For this review, take the finished solid that the model builds, in its own axes (mm). A direction names the side the tool comes from. Coordinates: 2 decimals unless noted, no trailing zeros. Loops run counter-clockwise (first coordinate to the right, second up) from the corner with the lowest first, then second, coordinate; pieces in that order, holes last. Notation, with made-up numbers: M 7,83 L 37,83 A20 ccw 37,94 Z; hole C 75.5,64.25 d1. An arc over 180 degrees is marked long. Write item = value, one per line.
from build123d import *

# Parameters (mm, degrees)
BOSS_EXTRUDE1_DEPTH = 25
SKETCH2_R           = 4
SKETCH2_R_2         = 1.5
CUT_EXTRUDE1_DEPTH  = 69.271516755
SKETCH3_R           = 4
SKETCH3_R_2         = 1.5
CUT_EXTRUDE2_DEPTH  = 71.774289117


with BuildPart() as part:
    # Sketch1 → Boss-Extrude1 (new body)
    with BuildSketch(Plane.XY):
        Polygon((-26, 30), (-26, -28), (26, -28), (26, 30), (28, 30), (28, -30), (-28, -30), (-28, 30), align=None)
    extrude(amount=BOSS_EXTRUDE1_DEPTH)

    # Sketch2 → Cut-Extrude1 (cut, through all)
    with BuildSketch(Plane(origin=(28, 0, 0), x_dir=(0, 0, -1), z_dir=(1, 0, 0))):
        with Locations((-12.5, 17.5)):
            Circle(SKETCH2_R)
        with Locations((-19.5, 17.5)):
            Circle(SKETCH2_R_2)
        with Locations((-12.5, -1.5)):
            Circle(SKETCH2_R_2)
        with Locations((-12.5, -18.5)):
            Circle(SKETCH2_R_2)
        with Locations((-12.5, 24.5)):
            Circle(SKETCH2_R_2)
        with Locations((-5.5, 17.5)):
            Circle(SKETCH2_R_2)
        with Locations((-12.5, 10.5)):
            Circle(SKETCH2_R_2)
        with BuildLine():
            Line((-25, 17.5), (-25, 33.655619926))
            Line((-25, 33.655619926), (0, 33.655619926))
            Line((0, 33.655619926), (0, 17.5))
            ThreePointArc((0, 17.5), (-12.5, 30), (-25, 17.5))
        make_face()
    extrude(amount=-CUT_EXTRUDE1_DEPTH, mode=Mode.SUBTRACT)

    # Sketch3 → Cut-Extrude2 (cut, through all)
    with BuildSketch(Plane.XZ.offset(30)):
        with Locations(Location((0, 12.5, 0), (0, 0, 270))):
            Circle(SKETCH3_R)
        with Locations(Location((-7, 12.5, 0), (0, 0, 270))):
            Circle(SKETCH3_R_2)
        with Locations(Location((0, 19.5, 0), (0, 0, 270))):
            Circle(SKETCH3_R_2)
        with Locations(Location((7, 12.5, 0), (0, 0, 270))):
            Circle(SKETCH3_R_2)
        with Locations(Location((0, 5.5, 0), (0, 0, 270))):
            Circle(SKETCH3_R_2)
        with Locations(Location((-19, 12.5, 0), (0, 0, 270))):
            Circle(SKETCH3_R_2)
        with Locations(Location((19, 12.5, 0), (0, 0, 270))):
            Circle(SKETCH3_R_2)
    extrude(amount=-CUT_EXTRUDE2_DEPTH, mode=Mode.SUBTRACT)


solid = part.part
Q1. For line 1 along X through (y, z) = (-28.55, 12.5); line 2 along Y through (x, z) = (-26.75, 12.5); line 3 along X through (y, z) = (10.5, 19.5), list the stretches that pass through material, from the lowest coordinate up.
Solved:
line_1 = -28 to -20.5, -17.5 to -8.5, -5.5 to -4, 4 to 5.5, 8.5 to 17.5, 20.5 to 28
line_2 = -30 to -20, -17 to -3, 0 to 9, 12 to 13.5, 21.5 to 23, 26 to 30
line_3 = -28 to -26, 26 to 28
Q2. Machinability: for faces 1 (the face through (27.014, 29.997, 12.225)), 2 (the face through (5, -28, 12)), which of the approach directions +Z, -Z, +X, -X, +Y, -Y give a long, thin tool a straight path to every point of the face, cutting with its end or side? Answer none if there is none.
Solved:
face_1 = +X, -X, +Y
face_2 = +Z, -Z, +Y
Q3. Draft analysis for pull direction X (two halves, no side actions). For faces 3 (the face through (-8.464, -29.014, 12.825)), 4 (the face through (27.01, -17.49, 13.61)), 5 (the face through (-28, 0, 10)), state which applies: +X half, -X half, draft (parallel to the pull), parting line (faces both ways), or undercut.
Solved:
face_3 = undercut
face_4 = draft
face_5 = -X half
Q4. Add section A-A (x = 0). Write out the cut boundary in (y, z), and give its area (3 significant figures).
Solved:
outline = M -30,0 L -28,0 L -28,4 L -30,4 Z; M -30,7 L -28,7 L -28,8.5 L -30,8.5 Z; M -30,16.5 L -28,16.5 L -28,18 L -30,18 Z; M -30,21 L -28,21 L -28,25 L -30,25 Z
area = 22.0 mm²
Q5. Add section C-C (x = -7). Write out the cut boundary in (y, z), and give its area (3 significant figures).
Solved:
outline = M -30,0 L -28,0 L -28,11 L -30,11 Z; M -30,14 L -28,14 L -28,25 L -30,25 Z
area = 44.0 mm²
Q6. Add section B-B (y = -14.5). Write out the cut boundary in (x, z).
Solved:
outline = M -28,0 L -26,0 L -26,25 L -28,25 Z; M 26,0 L 28,0 L 28,25 L 26,25 Z
Q7. For pin 1 Ø7.5 at (x, z) = (5.5, 12.5) entering from +Y; pin 2 Ø5 at (y, z) = (10.5, 12.5) entering from +X; pin 3 Ø2.5 at (x, z) = (0, 5.5) entering from -Y, all flat-tipped, find the tip position at first contact; note any pin that passes through.
Solved:
pin_1 = -28
pin_2 = 28
pin_3 = through
Q8. Add section D-D (y = 10.5). Write out the cut boundary in (x, z).
Solved:
outline = M -28,0 L -26,0 L -26,11 L -28,11 Z; M -28,14 L -26,14 L -26,25 L -28,25 Z; M 26,0 L 28,0 L 28,11 L 26,11 Z; M 26,14 L 28,14 L 28,25 L 26,25 Z
